The listing builds one solid part. Answer for the finished solid, in the listing's coordinates (mm). A direction names the side the tool comes from. Coordinates: 2 decimals unless noted, no trailing zeros. Write each loop counter-clockwise with the first axis right and the second up, starting at its lowest first coordinate (ties: lowest second). Pieces come first, ordered by that corner, then holes.
```python
from build123d import *

# Parameters (mm, degrees)
SKETCH1_R           = 1
BOSS_EXTRUDE1_DEPTH = 1.6
FILLET1_R           = 0.15
SKETCH2_R           = 1.5
CUT_EXTRUDE1_DEPTH  = 26.118429106
FILLET2_R           = 0.15
CUT_EXTRUDE2_DEPTH  = 0.5
FILLET3_R           = 0.1
FILLET4_R           = 0.15


with BuildPart() as part:
    # Sketch1 → Boss-Extrude1 (new body)
    with BuildSketch(Plane.XY):
        with BuildLine():
            Line((20.711831818, 0), (-7.714550435, 0))
            Line((-7.714550435, 0), (-8.64132713, -0.926776695))
            ThreePointArc((-8.64132713, -0.926776695), (-8.722432968, -0.980969883), (-8.818103826, -1))
            Line((-8.818103826, -1), (-16.964550435, -1))
            ThreePointArc((-16.964550435, -1), (-17.14132713, -0.926776695), (-17.214550435, -0.75))
            Line((-17.214550435, -0.75), (-17.214550435, 4.75))
            ThreePointArc((-17.214550435, 4.75), (-17.14132713, 4.926776695), (-16.964550435, 5))
            Line((-16.964550435, 5), (20.715695772, 5))
            ThreePointArc((20.715695772, 5), (20.782883317, 4.990802479), (20.845127191, 4.96388667))
            Line((20.845127191, 4.96388667), (24.443133824, 2.786588264))
            ThreePointArc((24.443133824, 2.786588264), (24.56367691, 2.576271817), (24.449189394, 2.362598581))
            Line((24.449189394, 2.362598581), (20.847318807, 0.039896988))
            ThreePointArc((20.847318807, 0.039896988), (20.782451386, 0.010181576), (20.711831818, 0))
        make_face()
        with Locations((-13.714550435, 2.2)):
            Circle(SKETCH1_R, mode=Mode.SUBTRACT)
    extrude(amount=BOSS_EXTRUDE1_DEPTH)

    # Fillet1
    fillet1_edges = [part.edges().sort_by_distance(p)[0] for p in [
        (20.782451386, 0.010181576, 1.6),
        (-8.722432968, -0.980969883, 0),
        (-12.89132713, -1, 0),
        (-17.14132713, -0.926776695, 0),
        (-17.214550435, 2, 0),
        (-17.14132713, 4.926776695, 0),
        (1.875572668, 5, 0),
        (20.782883317, 4.990802479, 0),
        (22.644130508, 3.875237467, 0),
        (24.56367691, 2.576271817, 0),
        (22.6482541, 1.201247785, 0),
        (22.6482541, 1.201247785, 1.6),
        (20.782451386, 0.010181576, 0),
        (6.498640691, 0, 0),
        (-8.177938783, -0.463388348, 0),
        (24.56367691, 2.576271817, 1.6),
        (22.644130508, 3.875237467, 1.6),
        (20.782883317, 4.990802479, 1.6),
        (1.875572668, 5, 1.6),
        (-17.14132713, 4.926776695, 1.6),
        (-17.214550435, 2, 1.6),
        (-17.14132713, -0.926776695, 1.6),
        (-12.89132713, -1, 1.6),
        (-8.177938783, -0.463388348, 1.6),
        (-8.722432968, -0.980969883, 1.6),
        (6.498640691, 0, 1.6),
    ]]
    fillet(fillet1_edges, radius=FILLET1_R)

    # Sketch2 → Cut-Extrude1 (cut, through all)
    with BuildSketch(Plane.XY.offset(1.6)):
        with Locations((20.727351555, 2.5)):
            Circle(SKETCH2_R)
    extrude(amount=-CUT_EXTRUDE1_DEPTH, mode=Mode.SUBTRACT)

    # Fillet2
    fillet2_edges = [part.edges().sort_by_distance(p)[0] for p in [
        (-14.714550435, 2.2, 0),
        (-14.714550435, 2.2, 1.6),
    ]]
    fillet(fillet2_edges, radius=FILLET2_R)

    # Sketch3 → Cut-Extrude2 (cut)
    with BuildSketch(Plane(origin=(0, 0, 0), x_dir=(-1, 0, 0), z_dir=(0, 0, -1))):
        with BuildLine():
            Line((-10.767468339, 4.35), (1.232531661, 4.35))
            ThreePointArc((1.232531661, 4.35), (-4.767468339, 3.428784028), (-10.767468339, 4.35))
        make_face()
    extrude(amount=-CUT_EXTRUDE2_DEPTH, mode=Mode.SUBTRACT)

    # Fillet3
    fillet3_edges = [part.edges().sort_by_distance(p)[0] for p in [
        (-1.232531661, 4.35, 0.25),
        (10.767468339, 4.35, 0.25),
    ]]
    fillet(fillet3_edges, radius=FILLET3_R)

    # Fillet4
    fillet4_edges = [part.edges().sort_by_distance(p)[0] for p in [
        (4.767468339, 3.428784028, 0),
        (4.767468339, 4.35, 0),
        (10.17544157, 4.263461428, 0),
        (-0.640504891, 4.263461428, 0),
    ]]
    fillet(fillet4_edges, radius=FILLET4_R)


solid = part.part
```
(1) This flat-tipped pin is pushed along its axis until it touches: pin 1 (1.8 mm diameter, centred on x = 20.73, y = 2.5, fed in from -Z). Where does it stop, or does it pass through?
(2) Section B-B, the plane x = -3.5 is taken. Write down the section's boundary in (y, z).
(3) Section A-A, the plane z = 1 is taken. Write down the section's boundary in (x, y), plus the area to 3 significant figures.
(4) Find the intervals of material crossed by probe 1 along X at (y, z) = (2, 0.7); probe 2 along Y at (x, z) = (-1, 0.4); probe 3 along Y at (x, z) = (21.5, 1), in increasing order.
(5) Which of the six approach directions +Z, -Z, +X, -X, +Y, -Y give full straight-line access (tool end or side, diameter ignored) to faces 1 (the flat face through (7, 0, 1)), 2 (the flat face through (4, 3, 0))?
(6) For a pull along Y with two mould halves and no side action, classify faces 3 (the flat face through (-17.215, 2, 1)), 4 (the flat face through (5, 4, 0.5)), 5 (the flat face through (-13, -1, 1)) as pulls with the +Y half, pulls with the -Y half, needs draft (parallel to the pull), parting line crosses it, or undercut.
Solution:
1. pin 1: passes through
2. outline: (0, 0.15) arc R0.15 ccw to (0.15, 0) - (4.85, 0) arc R0.15 ccw to (5, 0.15) - (5, 1.45) arc R0.15 ccw to (4.85, 1.6) - (0.15, 1.6) arc R0.15 ccw to (0, 1.45) - close
3. outline: (-17.21, -0.75) arc R0.25 ccw to (-16.96, -1) - (-8.82, -1) arc R0.25 ccw to (-8.64, -0.93) - (-7.71, 0) - (20.71, 0) arc R0.25 ccw to (20.85, 0.04) - (24.45, 2.36) arc R0.25 ccw to (24.44, 2.79) - (20.85, 4.96) arc R0.25 ccw to (20.72, 5) - (-16.96, 5) arc R0.25 ccw to (-17.21, 4.75) - close; hole circle Ø2 at (-13.71, 2.2); hole circle Ø3 at (20.73, 2.5)
3. area: 199 mm2
4. probe 1: x = -17.21 to -14.69, -12.73 to 19.31, 22.14 to 23.89
4. probe 2: y = 0 to 5
4. probe 3: y = 0.46 to 1.21, 3.79 to 4.57
5. face 1: +Z, -Z, +X, -Y
5. face 2: -Z, +X, -X, +Y, -Y
6. face 3: needs draft
6. face 4: undercut
6. face 5: pulls with the -Y half
